Part model, mm, in its own coordinate system. Face numbers are marked on the shaded views. A direction names the side the tool comes from. Round coordinates to 2 decimals unless told otherwise and drop trailing zeros. Write each loop counter-clockwise with the first axis right and the second up, starting at its lowest first coordinate (ties: lowest second). Pieces come first, ordered by that corner, then holes. Notation, with made-up numbers: M 79,68.5 L 90,68.5 A30 cw 90,91.5 Z; hole C 71.25,73.5 d11. An arc over 180 degrees is marked long. One line per question, with ' | ' between items. Start each with the question number.
1) Wall check: probe 1 along Z at (x, y) = (-0.25, 4.5); probe 2 along X at (y, z) = (7.75, 8.25); probe 3 along Z at (x, y) = (-2.75, 3.25). Give the ranges that are in metal, low to high. Write a range as [from, to].
2) Drop flat-ended pins along their axis: pin 1 Ø5 at (x, z) = (-4, 3.5) entering from -Y; pin 2 Ø0.8 at (x, z) = (-4, 8.5) entering from +Y; pin 3 Ø3 at (x, z) = (-3.5, 3) entering from +Y; pin 4 Ø1.2 at (x, y) = (-5.5, 7.5) entering from +Z. Give the stop position or say it passes through.
3) Mould opens along X. For the marked faces 1, 2, 3 and 4 say: pulls with the +X half, pulls with the -X half, needs draft (parallel to the pull), parting line crosses it, or undercut.
4) Tool access for the marked faces 5, 6 and 7: list every direction of +Z, -Z, +X, -X, +Y, -Y with a clear straight run to the whole face (end or side of a thin tool).
5) Saw through at B-B (x = 0). List the corners of the cut face in (y, z), plus the area to 3 significant figures.
6) Saw through at D-D (z = 4.5). List the corners of the cut face in (x, y), plus the area to 3 significant figures.
7) Saw through at A-A (z = 0). List the corners of the cut face in (x, y).
8) Saw through at C-C (y = 8.5). List the corners of the cut face in (x, z).
```python
from build123d import *

# Parameters (mm, degrees)
SKETCH1_W           = 24
SKETCH1_H           = 18
SKETCH1_R           = 6.4
BOSS_EXTRUDE1_DEPTH = 10
SKETCH2_W           = 22
SKETCH2_H           = 1
CUT_EXTRUDE1_DEPTH  = 4
SHELL1_DEPTH        = 8.9
SHELL1_2_DEPTH      = 4.9


# Read off the part's stored shape, not the designer's step: Shell1
with BuildPart() as part:
    # Sketch1 → Boss-Extrude1 (new body)
    with BuildSketch(Plane(origin=(0, 0, 0), x_dir=(1, 0, 0), z_dir=(0, 1, 0))):
        Rectangle(SKETCH1_W, SKETCH1_H)
        with Locations(Location((0, 0, 0), (0, 0, 270))):
            Circle(SKETCH1_R, mode=Mode.SUBTRACT)
    extrude(amount=BOSS_EXTRUDE1_DEPTH)

    # Sketch2 → Cut-Extrude1 (cut)
    with BuildSketch(Plane(origin=(0, 10, 0), x_dir=(1, 0, 0), z_dir=(0, 1, 0))):
        with Locations((0, 8.5)):
            Rectangle(SKETCH2_W, SKETCH2_H)
        with Locations((0, -8.5)):
            Rectangle(SKETCH2_W, SKETCH2_H)
    extrude(amount=-CUT_EXTRUDE1_DEPTH, mode=Mode.SUBTRACT)

    # Shell1 outline → Shell1 (cut)
    with BuildSketch(Plane(origin=(0, 0, 0), x_dir=(1, 0, 0), z_dir=(0, 1, 0))):
        with BuildLine():
            ThreePointArc((2.939387691, 6.9), (7.5, 0), (2.939387691, -6.9))
            Line((2.939387691, -6.9), (10.9, -6.9))
            Line((10.9, -6.9), (10.9, 6.9))
            Line((10.9, 6.9), (2.939387691, 6.9))
        make_face()
        with BuildLine():
            ThreePointArc((-2.939387691, -6.9), (-7.5, 0), (-2.939387691, 6.9))
            Line((-2.939387691, 6.9), (-10.9, 6.9))
            Line((-10.9, 6.9), (-10.9, -6.9))
            Line((-10.9, -6.9), (-2.939387691, -6.9))
        make_face()
    extrude(amount=SHELL1_DEPTH, mode=Mode.SUBTRACT)

    # Shell1 2 outline → Shell1 2 (cut)
    with BuildSketch(Plane(origin=(0, 0, 0), x_dir=(1, 0, 0), z_dir=(0, 1, 0))):
        with BuildLine():
            ThreePointArc((-2.939387691, 6.9), (0, 7.5), (2.939387691, 6.9))
            Line((2.939387691, 6.9), (10.9, 6.9))
            Line((10.9, 6.9), (10.9, 7.9))
            Line((10.9, 7.9), (-10.9, 7.9))
            Line((-10.9, 7.9), (-10.9, 6.9))
            Line((-10.9, 6.9), (-2.939387691, 6.9))
        make_face()
        with BuildLine():
            Line((10.9, -6.9), (2.939387691, -6.9))
            ThreePointArc((2.939387691, -6.9), (0, -7.5), (-2.939387691, -6.9))
            Line((-2.939387691, -6.9), (-10.9, -6.9))
            Line((-10.9, -6.9), (-10.9, -7.9))
            Line((-10.9, -7.9), (10.9, -7.9))
            Line((10.9, -7.9), (10.9, -6.9))
        make_face()
    extrude(amount=SHELL1_2_DEPTH, mode=Mode.SUBTRACT)


solid = part.part
```
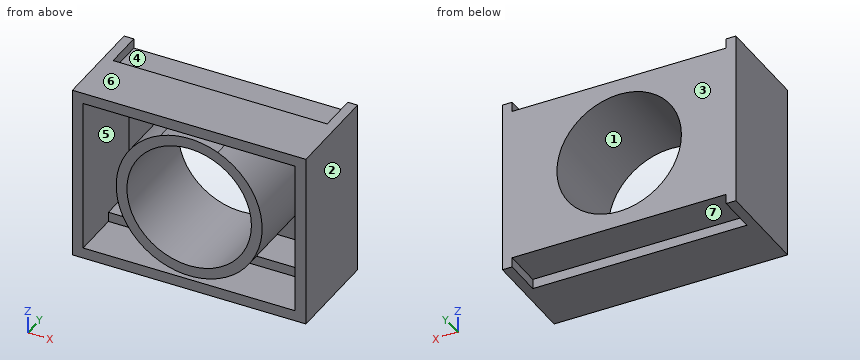
Answer key:
1) probe 1: z = [-9, -7.9], [-7.5, -6.4], [6.4, 7.5], [7.9, 9] | probe 2: x = [-12, -11], [11, 12] | probe 3: z = [-9, -7.9], [-6.98, -5.78], [5.78, 6.98], [7.9, 9]
2) pin 1: stops at y = 0 | pin 2: stops at y = 6 | pin 3: passes through | pin 4: stops at z = 8
3) face 1: undercut | face 2: pulls with the +X half | face 3: needs draft | face 4: undercut
4) face 5: -Y | face 6: +Z, +X, -X, +Y, -Y | face 7: -Z, +Y
5) outline: M 0,-9 L 6,-9 L 6,-8 L 10,-8 L 10,-6.4 L 0,-6.4 L 0,-7.5 L 4.9,-7.5 L 4.9,-7.9 L 0,-7.9 Z; M 0,6.4 L 10,6.4 L 10,8 L 6,8 L 6,9 L 0,9 L 0,7.9 L 4.9,7.9 L 4.9,7.5 L 0,7.5 Z | area: 40.1 mm2
6) outline: M -12,0 L -10.9,0 L -10.9,8.9 L -6,8.9 L -6,0 L -4.55,0 L -4.55,10 L -12,10 Z; M 4.55,0 L 6,0 L 6,8.9 L 10.9,8.9 L 10.9,0 L 12,0 L 12,10 L 4.55,10 Z | area: 61.8 mm2
7) outline: M -12,0 L -10.9,0 L -10.9,8.9 L -7.5,8.9 L -7.5,0 L -6.4,0 L -6.4,10 L -12,10 Z; M 6.4,0 L 7.5,0 L 7.5,8.9 L 10.9,8.9 L 10.9,0 L 12,0 L 12,10 L 6.4,10 Z
8) outline: M -12,-9 L -11,-9 L -11,-8 L 11,-8 L 11,-9 L 12,-9 L 12,9 L 11,9 L 11,8 L -11,8 L -11,9 L -12,9 Z; hole M -10.9,-6.9 L -2.94,-6.9 A7.5 cw -2.94,6.9 L -10.9,6.9 Z; hole C 0,0 d12.8; hole M 2.94,-6.9 L 10.9,-6.9 L 10.9,6.9 L 2.94,6.9 A7.5 cw Z
